from build123d import *

# Parameters (mm, degrees)
BOSS_EXTRUDE1_DEPTH = 7.5
SKETCH1_4_W         = 87
SKETCH1_4_H         = 2
BOSS_EXTRUDE2_DEPTH = 45
SKETCH2_R           = 1
CUT_EXTRUDE1_DEPTH  = 108.786826653


with BuildPart() as part:
    # Sketch1 → Boss-Extrude1 (new, symmetric)
    with BuildSketch(Plane(origin=(0, 0, 0), x_dir=(0, 0, -1), z_dir=(1, 0, 0))):
        Polygon((0, 0), (-7, 0), (-7, 50), (83, 50), (83, 52), (-9, 52), (-9, -2), (0, -2), align=None)
    extrude(amount=BOSS_EXTRUDE1_DEPTH, both=True)

    # Sketch1_4 → Boss-Extrude2 (add, symmetric)
    with BuildSketch(Plane(origin=(0, 0, 0), x_dir=(0, 0, -1), z_dir=(1, 0, 0))):
        with Locations((39.5, 51)):
            Rectangle(SKETCH1_4_W, SKETCH1_4_H)
    extrude(amount=BOSS_EXTRUDE2_DEPTH, both=True)

    # Sketch2 → Cut-Extrude1 (cut, through all)
    with BuildSketch(Plane(origin=(0, 0, 0), x_dir=(1, 0, 0), z_dir=(0, 1, 0))):
        with Locations(Location((-5.5, -3.5, 0), (0, 0, 270))):
            Circle(SKETCH2_R)
        with Locations(Location((5.5, -3.5, 0), (0, 0, 90))):
            Circle(SKETCH2_R)
    extrude(amount=-CUT_EXTRUDE1_DEPTH, mode=Mode.SUBTRACT)


solid = part.part
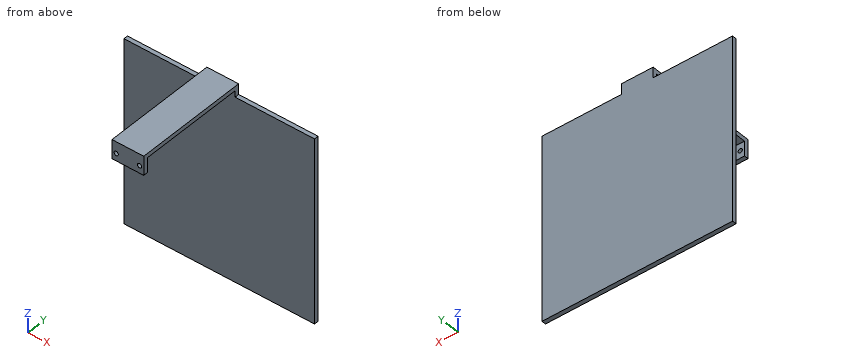
Here's how the part is built. I have some questions about the finished solid (model axes, mm). Give positions to 0.01 mm unless a question says otherwise; leave off trailing zeros. Order: outer loops, then holes, each group sorted by start corner. A loop starts at its lowest first (then second) coordinate and runs counter-clockwise, first axis right, second up. Notation, with made-up numbers: (79, -24) -> (118, -24) arc R33 ccw to (118, 5) -> close; hole circle Ø6 at (76.5, -6). An arc over 180 degrees is marked (long way). One line per item, written item: value. Start each with the question number.
1. Imagine slicing it at B-B, the plane z = -47. List the corners of the cut face in (x, y) for me, plus the area to 3 significant figures.
2. Will these pins go through, and if not, where does the flat tip stop? pin 1 Ø10 at (x, z) = (0, -22.5) entering from -Y; pin 2 Ø1 at (x, y) = (-27, 51.5) entering from +Z; pin 3 Ø1 at (x, y) = (-3.5, -0.5) entering from -Z.
3. Imagine slicing it at A-A, the plane y = 2. List the corners of the cut face in (x, z) for me.
4. I need wall thicknesses on probe 1 along X at (y, z) = (-0.7, 3.5); probe 2 along Z at (x, y) = (5.5, -1.15); probe 3 along X at (y, z) = (-1, 3). Which ranges of each line are inside material? Lowest first, please. Write a range as from..to.
Values follow:
1. outline: (-45, 50) -> (45, 50) -> (45, 52) -> (-45, 52) -> close
1. area: 180 mm2
2. pin 1: stops at y = 50
2. pin 2: stops at z = 4
2. pin 3: stops at z = 0
3. outline: (-7.5, 7) -> (7.5, 7) -> (7.5, 9) -> (-7.5, 9) -> close
4. probe 1: x = -7.5..-6.5, -4.5..4.5, 6.5..7.5
4. probe 2: z = 0..2.5, 4.5..9
4. probe 3: x = -7.5..-6.37, -4.63..4.63, 6.37..7.5
